Source: CAD feature listing. Evaluate the final solid. Frame: model axes, mm. A direction names the side the tool comes from. Round coordinates to 2 decimals unless told otherwise and drop trailing zeros. Loops run counter-clockwise (first coordinate to the right, second up) from the corner with the lowest first, then second, coordinate; pieces in that order, holes last. Notation, with made-up numbers: (23, -6.5) -> (37, -6.5) arc R15 cw to (37, 0.5) -> close; hole circle Ø10 at (79, 28.25). An arc over 180 degrees is marked (long way). Put each result on its own line as item: value. Start each with the question number.
1. Cut plane B-B (z = 99). Return the cut outline in (x, y), then the cut area to 3 significant figures.
2. Cut plane A-A (x = 19). Return the cut outline in (y, z).
3. Cut plane C-C (x = 0). Return the cut outline in (y, z), then the cut area to 3 significant figures.
4. Set-up query: faces 5 (the flat face through (11.5, 0, 135)), 6 (the cylindrical face through (-31.861, 5.995, 69.389)). Return all of +Z, -Z, +X, -X, +Y, -Y with unobstructed straight access to the full face (end or side cutting, diameter ignored); none if empty.
5. Contact query for flat-ended pins moving along their axis: pin 1 (5.5 mm diameter, centred on x = -0.5, z = 135.5, fed in from +Y); pin 2 (5.5 mm diameter, centred on x = -19.5, z = 135.5, fed in from -Y); pin 3 (2.5 mm diameter, centred on x = 16.5, z = 135, fed in from -Y); pin 4 (8 mm diameter, centred on x = 4, y = -3.5, fed in from +Z). Output: stop coordinate, or through.
6. Draft query along X for faces 1 (the cylindrical face through (-31.861, -5.995, 69.389)), 2 (the flat face through (0, 0, 132)), 3 (the flat face through (18, -2.5, 135)), 4 (the cylindrical face through (-0.37, 6.75, 1.43)). Return one class per face: pulls with the +X half, pulls with the -X half, needs draft (parallel to the pull), parting line crosses it, or undercut.
7. Material intervals for L1, parallel to X at y = -1.25, z = 35; L2, parallel to Z at x = -27, y = 5; L3, parallel to X at y = -4.5, z = 127, sorted ascending.
```python
from build123d import *

# Parameters (mm, degrees)
ESQUISSE1_W             = 68
ESQUISSE1_H             = 16.5
BOSS_EXTRU_1_DEPTH      = 137
CONG_1_R                = 7.5
CONG_2_R                = 5
ESQUISSE2_W             = 12.5
ESQUISSE2_H             = 5
ENL_V_MAT_EXTRU_1_DEPTH = 5
CONG_3_R                = 1


with BuildPart() as part:
    # Esquisse1 → Boss.-Extru.1 (new body)
    with BuildSketch(Plane.XY):
        Rectangle(ESQUISSE1_W, ESQUISSE1_H)
    extrude(amount=BOSS_EXTRU_1_DEPTH)

    # Congé1
    cong_1_edges = [part.edges().sort_by_distance(p)[0] for p in [
        (-34, 8.25, 68.5),
        (34, 8.25, 68.5),
        (34, -8.25, 68.5),
        (-34, -8.25, 68.5),
    ]]
    fillet(cong_1_edges, radius=CONG_1_R)

    # Congé2
    cong_2_edges = [part.edges().sort_by_distance(p)[0] for p in [
        (34, 0, 0),
        (34, 0, 137),
        (-34, 0, 0),
        (0, 8.25, 0),
        (0, -8.25, 0),
        (-31.803300859, 6.053300859, 0),
        (-31.803300859, -6.053300859, 0),
        (31.803300859, 6.053300859, 0),
        (31.803300859, -6.053300859, 0),
        (0, -8.25, 137),
        (-34, 0, 137),
        (0, 8.25, 137),
        (-31.803300859, 6.053300859, 137),
        (-31.803300859, -6.053300859, 137),
        (31.803300859, 6.053300859, 137),
        (31.803300859, -6.053300859, 137),
    ]]
    fillet(cong_2_edges, radius=CONG_2_R)

    # Esquisse2 → Enlèv. mat.-Extru.1 (cut)
    with BuildSketch(Plane.XY.offset(137)):
        Polygon((-12.75, 1.5), (-22.75, 1.5), (-22.75, 0), (-19.52732972, -1.5), (-15.97267028, -1.5), (-12.75, 0), align=None)
        with BuildLine():
            Line((5, 1.5), (-5, 1.5))
            ThreePointArc((-5, 1.5), (-6.5, 0), (-5, -1.5))
            Line((-5, -1.5), (5, -1.5))
            ThreePointArc((5, -1.5), (6.5, 0), (5, 1.5))
        make_face()
        with Locations((17.75, 0)):
            Rectangle(ESQUISSE2_W, ESQUISSE2_H)
    extrude(amount=-ENL_V_MAT_EXTRU_1_DEPTH, mode=Mode.SUBTRACT)

    # Congé3
    # the kernel refuses this fillet: 1 mm, written as the material it adds along each edge
    with BuildSketch(Plane(origin=(-15.97267028, -1.5, 137), x_dir=(0.9066045100812768, 0.4219813530243817, 0), z_dir=(0, 0, -1)), Plane(origin=(-19.52732972, -1.5, 137), x_dir=(1, 0, 0), z_dir=(0, 0, -1))) as cong_3_piece_1:
        with BuildLine():
            CenterArc((CONG_3_R * 0.221326106591, -CONG_3_R), CONG_3_R, 90, 24.959741925)
            Line((-CONG_3_R * 0.200655246434, -CONG_3_R * 0.0933954899187), (0, 0))
            Line((0, 0), (CONG_3_R * 0.221326106591, 0))
        make_face()
    extrude(amount=5.553315266)
    with BuildSketch(Plane(origin=(-22.75, 0, 137), x_dir=(0.9066045100812758, -0.42198135302438383, 0), z_dir=(0, 0, -1))) as cong_3_piece_2:
        with BuildLine():
            CenterArc((CONG_3_R * 0.637564274773, -CONG_3_R), CONG_3_R, 90, 65.040258075)
            Line((-CONG_3_R * 0.269040235309, -CONG_3_R * 0.578018646976), (0, 0))
            Line((0, 0), (CONG_3_R * 0.637564274773, 0))
        make_face()
    extrude(amount=6.593910687)
    with BuildSketch(Plane(origin=(-22.75, 1.5, 137), x_dir=(0, -1, 0), z_dir=(0, 0, -1)), Plane(origin=(-12.75, 1.5, 137), x_dir=(-1, 0, 0), z_dir=(0, 0, -1))) as cong_3_piece_3:
        with BuildLine():
            CenterArc((CONG_3_R, -CONG_3_R), CONG_3_R, 90, 90)
            Line((0, -CONG_3_R), (0, 0))
            Line((0, 0), (CONG_3_R, 0))
        make_face()
    extrude(amount=7.5)
    with BuildSketch(Plane(origin=(-12.75, 0, 137), x_dir=(-0.906604510081276, -0.4219813530243839, 0), z_dir=(0, 0, -1))) as cong_3_piece_4:
        with BuildLine():
            CenterArc((CONG_3_R * 0.637564274773, CONG_3_R), CONG_3_R, 204.959741925, 65.040258075)
            Line((-CONG_3_R * 0.269040235309, CONG_3_R * 0.578018646976), (0, 0))
            Line((0, 0), (CONG_3_R * 0.637564274773, 0))
        make_face()
    extrude(amount=6.593910687)


solid = part.part
```
Solution:
1. outline: (-34, -0.75) arc R7.5 ccw to (-26.5, -8.25) -> (26.5, -8.25) arc R7.5 ccw to (34, -0.75) -> (34, 0.75) arc R7.5 ccw to (26.5, 8.25) -> (-26.5, 8.25) arc R7.5 ccw to (-34, 0.75) -> close
1. area: 1,070 mm^2
2. outline: (-8.25, 5) arc R5 ccw to (-3.25, 0) -> (3.25, 0) arc R5 ccw to (8.25, 5) -> (8.25, 132) arc R5 ccw to (3.25, 137) -> (2.5, 137) -> (2.5, 132) -> (-2.5, 132) -> (-2.5, 137) -> (-3.25, 137) arc R5 ccw to (-8.25, 132) -> close
3. outline: (-8.25, 5) arc R5 ccw to (-3.25, 0) -> (3.25, 0) arc R5 ccw to (8.25, 5) -> (8.25, 132) arc R5 ccw to (3.25, 137) -> (1.5, 137) -> (1.5, 132) -> (-1.5, 132) -> (-1.5, 137) -> (-3.25, 137) arc R5 ccw to (-8.25, 132) -> close
3. area: 2,220 mm^2
4. face 5: +Z
4. face 6: +Z, -Z, -X, +Y
5. pin 1: stops at y = 8.19
5. pin 2: stops at y = -8.19
5. pin 3: stops at y = -7.93
5. pin 4: stops at z = 137
6. face 1: pulls with the -X half
6. face 2: undercut
6. face 3: undercut
6. face 4: needs draft
7. L1: x = -33.98 to 33.98
7. L2: z = 0.33 to 136.67
7. L3: x = -33 to 33
